Geometry check sheet. Reference: the model listing, model coordinates, mm. A direction names the side the tool comes from. Round coordinates to 2 decimals unless told otherwise and drop trailing zeros. Loops run counter-clockwise (first coordinate to the right, second up) from the corner with the lowest first, then second, coordinate; pieces in that order, holes last. Notation, with made-up numbers: M -34.5,21.5 L -8.5,21.5 A21 ccw -8.5,32.5 Z; hole C -21,-36 d8. An arc over 180 degrees is marked long. Use one line per item in the form item = value. Start each with the question number.
1. Cross-section at A-A (x = 13). Record the boundary of the cut face in (y, z), then the cut area to 3 significant figures.
2. Cross-section at B-B (y = 0). Record the boundary of the cut face in (x, z), then the cut area to 3 significant figures.
3. Set-up check for faces 4 (the flat face through (0, -67.5, 17)), 5 (the flat face through (24.875, -47, 22)), 6 (the flat face through (15, 9, 15)), 7 (the flat face through (0, -25, 23.964)), 8 (the flat face through (7.5, -25, 17)): record each of +Z, -Z, +X, -X, +Y, -Y from which the full face is reachable in a straight line by a thin tool's end or side.
4. Material ranges on line 1 (X direction, y = -30, z = 14); line 2 (X direction, y = -43, z = 30); line 3 (Y direction, x = 0, z = 5.5), recorded low to high.
5. Cross-section at D-D (z = 36.5). Record the boundary of the cut face in (x, y), then the cut area to 3 significant figures.
6. Go/stop test with flat-tipped pins: pin 1 (7.5 mm diameter, centred on y = 1.5, z = 11, fed in from +X); pin 2 (24 mm diameter, centred on y = 0, z = 15.01, fed in from -X); pin 3 (6 mm diameter, centred on x = -25, y = -38, fed in from +Z). Record where each tip stops, or that it passes through.
7. Draft check along Y on faces 1 (the flat face through (-7.5, -25, 16)), 2 (the flat face through (0, 12.5, 15)), 3 (the flat face through (0, 0, 30)). Enter one of: pulls with the +Y half, pulls with the -Y half, needs draft (parallel to the pull), parting line crosses it, or undercut.
8. Cross-section at C-C (z = 27). Record the boundary of the cut face in (x, y).
Autodesk Inventor part; units mm, degrees
ref_plane "YZ Plane" through (0, 0, 0) normal (1, 0, 0) x (0, 1, 0)
ref_plane "XZ Plane" through (0, 0, 0) normal (0, 1, 0) x (-1, 0, 0)
ref_plane "XY Plane" through (0, 0, 0) normal (0, 0, 1) x (1, 0, 0)
sketch "Sketch1" plane through (0, 0, 0) normal (0, 0, 1) x (1, 0, 0)
  line L0 (-15, 12.5) -> (15, 12.5)
  line L1 (15, 12.5) -> (15, -12.5)
  line L2 (15, -12.5) -> (-15, -12.5)
  line L3 (-15, -12.5) -> (-15, 12.5)
  line L4 (-15, 12.5) -> (15, -12.5) construction
  line L5 (15, 12.5) -> (-15, -12.5) construction
  point P0 (0, 0)
  dimension "d0" = 30
  dimension "d1" = 25
extrude "Extrusion1" add sketch "Sketch1" along normal blind 30
sketch "Sketch2" plane through (15, -12.5, 0) normal (1, 0, 0) x (0, 0, -1)
  circle A0 centre (-15.0077, 12.5) radius 7.5
  point P0 (0, 12.5)
  dimension "d4" = 15
extrude "Extrusion2" cut sketch "Sketch2" against normal through all
sketch "Sketch3" plane through (-15, -12.5, 0) normal (0, -1, 0) x (1, 0, 0)
  line L0 (7.5, 23.9638) -> (22.5, 23.9638)
  line L1 (22.5, 23.9638) -> (22.5, 8.9638)
  line L2 (22.5, 8.9638) -> (7.5, 8.9638)
  line L3 (7.5, 8.9638) -> (7.5, 23.9638)
  line L4 (7.5, 23.9638) -> (22.5, 8.9638) construction
  line L5 (22.5, 23.9638) -> (7.5, 8.9638) construction
  point P0 (15, 0)
  point P1 (15, 16.4638)
  dimension "d7" = 15
  dimension "d8" = 15
extrude "Extrusion3" add sketch "Sketch3" along normal blind 25
sketch "Sketch4" plane through (-15, -37.5, 0) normal (0, -1, 0) x (1, 0, 0)
  line L0 (-0.1247, 34.0483) -> (29.8753, 34.0483)
  line L1 (29.8753, 34.0483) -> (29.8753, -0.9517)
  line L2 (29.8753, -0.9517) -> (-0.1247, -0.9517)
  line L3 (-0.1247, -0.9517) -> (-0.1247, 34.0483)
  line L4 (-0.1247, 34.0483) -> (29.8753, -0.9517) construction
  line L5 (29.8753, 34.0483) -> (-0.1247, -0.9517) construction
  point P0 (15, 0)
  point P1 (14.8753, 16.5483)
  dimension "d11" = 30
  dimension "d12" = 35
extrude "Extrusion4" add sketch "Sketch4" along normal blind 30
sketch "Sketch5" plane through (-15.1247, -37.5, -0.9517) normal (-1, 0, 0) x (0, 0, 1)
  circle A0 centre (17.4156, -15.0883) radius 7.5
  point P0 (0.9517, 37.5)
  dimension "d15" = 15
extrude "Extrusion5" add sketch "Sketch5" along normal blind 10
sketch "Sketch6" plane through (14.8753, -37.5, 34.0483) normal (1, 0, 0) x (0, 0, -1)
  circle A0 centre (17.5844, -15.0883) radius 7.5
  circle A1 centre (17.5844, -15.0883) radius 7.5
  point P0 (34.0483, 37.5)
extrude "Extrusion6" add sketch "Sketch6" along normal blind 10
sketch "Sketch7" plane through (-25.1247, -52.5883, 16.4638) normal (-1, 0, 0) x (0, 0, 1)
  line L0 (-17.4156, -14.9117) -> (17.5844, -14.9117)
  circle A0 centre (0, 0) radius 23.0558
  point P0 (-16.4638, 52.5883)
extrude "Extrusion7" add sketch "Sketch7" along normal blind 10
sketch "Sketch8" plane through (24.8753, -52.5883, 16.4638) normal (1, 0, 0) x (0, 0, -1)
  circle A0 centre (0, 0) radius 7.5
  circle A1 centre (0, 0) radius 23.0558
  circle A2 centre (0, 0) radius 23.056
  point P0 (16.4638, 52.5883)
  dimension "d22" = 46.112
extrude "Extrusion8" add sketch "Sketch8" along normal blind 10 contours A0 | A1
properties part number "Part4_remodified"
Reported:
q1.outline = M -67.5,-0.95 L -37.5,-0.95 L -37.5,34.05 L -67.5,34.05 Z; M -12.5,0 L 12.5,0 L 12.5,30 L -12.5,30 Z; hole C 0,15.01 d15
q1.area = 1,620 mm²
q2.outline = M -15,0 L 15,0 L 15,7.51 L -15,7.51 Z; M -15,22.51 L 15,22.51 L 15,30 L -15,30 Z
q2.area = 450 mm²
q3.face_4 = +Z, -Z, -Y
q3.face_5 = none
q3.face_6 = +Z, -Z, +X, +Y
q3.face_7 = +Z
q3.face_8 = +Z, -Z
q4.line_1 = -35.12 to -25.12, -7.5 to 7.5, 24.88 to 34.88
q4.line_2 = -35.12 to -25.12, -15.12 to 14.88, 24.88 to 34.88
q4.line_3 = -67.5 to -37.5, -12.5 to 12.5
q5.outline = M -35.12,-64 L -25.12,-64 L -25.12,-41.18 L -35.12,-41.18 Z; M 24.88,-64 L 34.88,-64 L 34.88,-41.18 L 24.88,-41.18 Z
q5.area = 456 mm²
q6.pin_1 = 15
q6.pin_2 = -15
q6.pin_3 = 36.39
q7.face_1 = undercut
q7.face_2 = pulls with the +Y half
q7.face_3 = needs draft
q8.outline = M -35.12,-73.1 L -25.12,-73.1 L -25.12,-32.08 L -35.12,-32.08 Z; M -15.12,-67.5 L 14.88,-67.5 L 14.88,-37.5 L -15.12,-37.5 Z; M -15,-12.5 L 15,-12.5 L 15,12.5 L -15,12.5 Z; M 24.88,-73.1 L 34.88,-73.1 L 34.88,-32.08 L 24.88,-32.08 Z
